```python
from build123d import *

# Parameters (mm, degrees)
CROQUIS1_R              = 25.4
SALIENTE_EXTRUIR2_DEPTH = 10
CROQUIS4_R              = 14
CORTAR_EXTRUIR2_DEPTH   = 47
CROQUIS5_R              = 25.4
CROQUIS5_R_2            = 22.5
CORTAR_EXTRUIR4_DEPTH   = 7
CROQUIS6_R              = 1.35
CORTAR_EXTRUIR5_DEPTH   = 37


with BuildPart() as part:
    # Croquis1 → Saliente-Extruir2 (new body)
    with BuildSketch(Plane(origin=(0, 0, 0), x_dir=(1, 0, 0), z_dir=(0, 1, 0))):
        Circle(CROQUIS1_R)
    extrude(amount=SALIENTE_EXTRUIR2_DEPTH)

    # Croquis4 → Cortar-Extruir2 (cut)
    with BuildSketch(Plane(origin=(0, 0, 0), x_dir=(1, 0, 0), z_dir=(0, 1, 0))):
        Circle(CROQUIS4_R)
    extrude(amount=CORTAR_EXTRUIR2_DEPTH, mode=Mode.SUBTRACT)

    # Croquis5 → Cortar-Extruir4 (cut)
    with BuildSketch(Plane(origin=(0, 0, 0), x_dir=(1, 0, 0), z_dir=(0, 1, 0))):
        Circle(CROQUIS5_R)
        Circle(CROQUIS5_R_2, mode=Mode.SUBTRACT)
    extrude(amount=CORTAR_EXTRUIR4_DEPTH, mode=Mode.SUBTRACT)

    # Croquis6 → Cortar-Extruir5 (cut)
    with BuildSketch(Plane(origin=(0, 0, 0), x_dir=(1, 0, 0), z_dir=(0, 1, 0))):
        with Locations((24, 0)):
            Circle(CROQUIS6_R)
        with Locations((-12, -20.784609691)):
            Circle(CROQUIS6_R)
        with Locations((-12, 20.784609691)):
            Circle(CROQUIS6_R)
    extrude(amount=CORTAR_EXTRUIR5_DEPTH, mode=Mode.SUBTRACT)


solid = part.part
```
Design review of the part built by this model. Coordinates are the model's own, in mm. Coordinates: 2 decimals unless noted, no trailing zeros. Loops run counter-clockwise (first coordinate to the right, second up) from the corner with the lowest first, then second, coordinate; pieces in that order, holes last. Notation, with made-up numbers: M 40,-14.5 L 50,-14.5 A16 cw 50,6.5 Z; hole C -39,8.25 d5. An arc over 180 degrees is marked long. One line per question, with ' | ' between items.
(1) Draft analysis for pull direction Z (two halves, no side actions). For faces 1 (the face through (-10, 7, 21)), 2 (the face through (10.382, 3.451, 19.961)), 3 (the face through (24.62, 8.48, 1.2)), state which applies: released by +Z, released by -Z, zero draft, split by the parting line, or undercut.
Filled in:
face 1: zero draft | face 2: split by the parting line | face 3: undercut
(2) We need section B-B (x = -7.5). Give the boundary of the cut face in (y, z).
Filled in:
outline: M 0,-21.21 L 7,-21.21 L 7,-24.27 L 10,-24.27 L 10,-11.82 L 0,-11.82 Z; M 0,11.82 L 10,11.82 L 10,24.27 L 7,24.27 L 7,21.21 L 0,21.21 Z
(3) Wall thickness on probe 1 along X at (y, z) = (5.5, 0); probe 2 along Z at (x, y) = (0.5, 8): over which ranges is each line inside the solid? List them lowest first.
Filled in:
probe 1: x = -22.5 to -14, 14 to 22.5 | probe 2: z = -25.4 to -13.99, 13.99 to 25.4
(4) For pin 1 Ø4 at (y, z) = (2, -19.5) entering from -X; pin 2 Ø1.5 at (x, y) = (-3.5, 6.5) entering from +Z; pin 3 Ø1 at (x, y) = (10, 5) entering from +Z, all flat-tipped, find the tip position at first contact; note any pin that passes through.
Filled in:
pin 1: stops at x = -14.14 | pin 2: stops at z = 25.23 | pin 3: stops at z = 20.4
(5) We need section C-C (z = 15). Give the boundary of the cut face in (x, y).
Filled in:
outline: M -20.5,7 L -16.77,7 L -16.77,0 L 16.77,0 L 16.77,7 L 20.5,7 L 20.5,10 L -20.5,10 Z
(6) We need section D-D (y = 5.25). Give the boundary of the cut face in (x, z), and give its area (3 significant figures).
Filled in:
outline: C 0,0 d45; hole C 0,0 d28 | area: 975 mm^2
(7) We need section A-A (z = 0). Give the boundary of the cut face in (x, y).
Filled in:
outline: M -25.4,7 L -22.5,7 L -22.5,0 L -14,0 L -14,10 L -25.4,10 Z; M 14,0 L 22.5,0 L 22.5,7 L 22.65,7 L 22.65,10 L 14,10 Z; M 25.35,7 L 25.4,7 L 25.4,10 L 25.35,10 Z
